Design review of the part built by this model. Coordinates are the model's own, in mm. Round coordinates to 2 decimals unless told otherwise and drop trailing zeros. Order: outer loops, then holes, each group sorted by start corner. A loop starts at its lowest first (then second) coordinate and runs counter-clockwise, first axis right, second up. Notation, with made-up numbers: (-16, -11.75) - (1, -11.75) arc R22 cw to (1, 12.25) - close; hole circle Ø10 at (72.5, -29.5). An arc over 180 degrees is marked (long way). Write item = value, one per line.
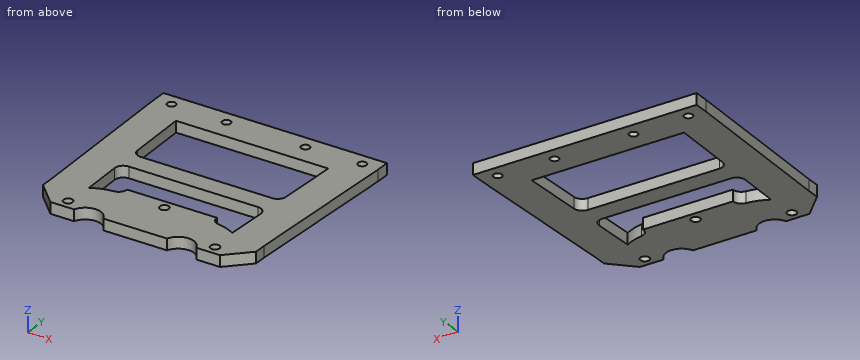
from build123d import *

# Parameters (mm, degrees)
SKETCH1_R           = 1.610311209
SKETCH1_R_2         = 1.5
BOSS_EXTRUDE1_DEPTH = 4
FILLET1_R           = 3


with BuildPart() as part:
    # Sketch1 → Boss-Extrude1 (new body)
    with BuildSketch(Plane.XY):
        with BuildLine():
            Line((-38.110698604, 1.610311209), (-30.354366282, -6.146021113))
            Line((-30.354366282, -6.146021113), (-21.854366282, -6.146021113))
            ThreePointArc((-21.854366282, -6.146021113), (-16.639882489, -2.482124138), (-11.425398696, -6.146021113))
            Line((-11.425398696, -6.146021113), (11.425398696, -6.146021113))
            ThreePointArc((11.425398696, -6.146021113), (16.639882489, -2.482124138), (21.854366282, -6.146021113))
            Line((21.854366282, -6.146021113), (30.354366282, -6.146021113))
            Line((30.354366282, -6.146021113), (38.110698604, 1.610311209))
            Line((38.110698604, 1.610311209), (38.110698604, 5.904474432))
            Line((38.110698604, 5.904474432), (40, 64.661867252))
            Line((40, 64.661867252), (40, 69.661867252))
            Line((40, 69.661867252), (-40, 69.661867252))
            Line((-40, 69.661867252), (-40, 64.661867252))
            Line((-40, 64.661867252), (-38.110698604, 5.904474432))
            Line((-38.110698604, 5.904474432), (-38.110698604, 1.610311209))
        make_face()
        with Locations((0, 9.661867252)):
            Circle(SKETCH1_R, mode=Mode.SUBTRACT)
        with Locations((-26.301749741, -2.683852014)):
            Circle(SKETCH1_R, mode=Mode.SUBTRACT)
        with Locations((26.301749741, -2.683852014)):
            Circle(SKETCH1_R, mode=Mode.SUBTRACT)
        with Locations((34.124535685, 65.161867252)):
            Circle(SKETCH1_R_2, mode=Mode.SUBTRACT)
        with Locations((14.124535685, 64.661867252)):
            Circle(SKETCH1_R_2, mode=Mode.SUBTRACT)
        with Locations((-14.124535685, 64.661867252)):
            Circle(SKETCH1_R_2, mode=Mode.SUBTRACT)
        with Locations((-34.124535685, 65.161867252)):
            Circle(SKETCH1_R_2, mode=Mode.SUBTRACT)
        Polygon((-27.252382744, 57.161867252), (-26.45560174, 32.381927681), (26.45560174, 32.381927681), (27.252382744, 57.161867252), align=None, mode=Mode.SUBTRACT)
        with BuildLine():
            Line((25.658820737, 7.60198811), (26.230521812, 25.381927681))
            Line((26.230521812, 25.381927681), (-26.230521812, 25.381927681))
            Line((-26.230521812, 25.381927681), (-25.658820737, 7.60198811))
            ThreePointArc((-25.658820737, 7.60198811), (-20.760848223, 9.540954041), (-15.511590599, 9.98256249))
            Line((-15.511590599, 9.98256249), (-15.511590599, 12.98256249))
            Line((-15.511590599, 12.98256249), (16.639882489, 12.98256249))
            Line((16.639882489, 12.98256249), (16.639882489, 10.017875862))
            ThreePointArc((16.639882489, 10.017875862), (21.308334072, 9.403441757), (25.658820737, 7.60198811))
        make_face(mode=Mode.SUBTRACT)
    extrude(amount=BOSS_EXTRUDE1_DEPTH)

    # Fillet1
    fillet1_edges = [part.edges().sort_by_distance(p)[0] for p in [
        (-26.45560174, 32.381927681, 2),
        (26.45560174, 32.381927681, 2),
        (-26.230521812, 25.381927681, 2),
        (-15.511590599, 9.98256249, 2),
        (16.639882489, 10.017875862, 2),
        (26.230521812, 25.381927681, 2),
    ]]
    fillet(fillet1_edges, radius=FILLET1_R)


solid = part.part
1) We need section D-D on y = 29. Write out the cut boundary in (x, z), and give its area (3 significant figures).
Findings:
outline = (-38.85, 0) - (38.85, 0) - (38.85, 4) - (-38.85, 4) - close
area = 311 mm^2
2) To check wall thickness, follow L1, parallel to Y at x = 16.5, z = 1.85; L2, parallel to Y at x = 7.5, z = 3.4; L3, parallel to Y at x = 0, z = 2.7. State the ranges of each line that lie inside material, in increasing order. Write a range as from..to.
Findings:
L1 = -2.48..12.98, 25.38..32.38, 57.16..69.66
L2 = -6.15..12.98, 25.38..32.38, 57.16..69.66
L3 = -6.15..8.05, 11.27..12.98, 25.38..32.38, 57.16..69.66
3) We need section B-B on y = 45. Write out the cut boundary in (x, z).
Findings:
outline = (-39.37, 0) - (-26.86, 0) - (-26.86, 4) - (-39.37, 4) - close; (26.86, 0) - (39.37, 0) - (39.37, 4) - (26.86, 4) - close
4) We need section C-C on z = 1.3. Give the number of separate pieces and of enclosed holes in the cut face, and give its area (3 significant figures).
Findings:
separate_pieces = 1
enclosed_holes = 9
area = 3,700 mm^2
5) We need section A-A on x = 0. Write out the cut boundary in (y, z).
Findings:
outline = (-6.15, 0) - (8.05, 0) - (8.05, 4) - (-6.15, 4) - close; (11.27, 0) - (12.98, 0) - (12.98, 4) - (11.27, 4) - close; (25.38, 0) - (32.38, 0) - (32.38, 4) - (25.38, 4) - close; (57.16, 0) - (69.66, 0) - (69.66, 4) - (57.16, 4) - close
